from build123d import *

# Parameters (mm, degrees)
BOSS_EXTRUDE1_DEPTH     = 40
SKETCH2_W               = 26
SKETCH2_H               = 6
CUT_EXTRUDE1_DEPTH      = 243.400412541
CUT_EXTRUDE1_DEPTH_BACK = 243.400412541
SKETCH4_R               = 2.5
CUT_EXTRUDE3_START      = 7.142108
SKETCH7_R               = 5
CUT_EXTRUDE3_DEPTH      = 54.857892


with BuildPart() as part:
    # Sketch1 → Boss-Extrude1 (new body)
    with BuildSketch(Plane.XY):
        with BuildLine():
            Line((0, 0), (228.6, 0))
            Line((228.6, 0), (228.6, 70))
            ThreePointArc((228.6, 70), (114.3, 23.006536612), (0, 70))
            Line((0, 70), (0, 0))
        make_face()
    extrude(amount=BOSS_EXTRUDE1_DEPTH)

    # Sketch2 → Cut-Revolve1 (revolve, cut)
    with BuildSketch(Plane(origin=(114.3, 0, 0), x_dir=(0, 0, -1), z_dir=(1, 0, 0))):
        with Locations((-20, 12.006536612)):
            Rectangle(SKETCH2_W, SKETCH2_H)
    revolve(axis=Axis((114.3, 185.506536612, 40), (0, 0, 1)), mode=Mode.SUBTRACT)

    # Sketch4 → Cut-Extrude1 (cut, two sides: drawn at the far end of the back side and taken through both)
    with BuildSketch(Plane.XZ.offset(-CUT_EXTRUDE1_DEPTH_BACK)):
        with Locations(Location((12.7, 20, 0), (0, 0, 270))):
            Circle(SKETCH4_R)
        with Locations(Location((215.9, 20, 0), (0, 0, 270))):
            Circle(SKETCH4_R)
    extrude(amount=CUT_EXTRUDE1_DEPTH + CUT_EXTRUDE1_DEPTH_BACK, mode=Mode.SUBTRACT)

    # Sketch7 → Cut-Extrude3 (cut)
    with BuildSketch(Plane(origin=(0, 70, 0), x_dir=(-1, 0, 0), z_dir=(0, -1, 0)).offset(CUT_EXTRUDE3_START)):
        with Locations(Location((-215.9, -20, 0), (0, 0, 270))):
            Circle(SKETCH7_R)
        with Locations(Location((-12.7, -20, 0), (0, 0, 270))):
            Circle(SKETCH7_R)
    extrude(amount=CUT_EXTRUDE3_DEPTH, mode=Mode.SUBTRACT)

    # Sketch9 → Cut-Revolve3 (revolve, cut)
    with BuildSketch(Plane(origin=(114.3, 0, 0), x_dir=(0, 0, -1), z_dir=(1, 0, 0))):
        Polygon((0, 18.806536612), (0, 23.006536612), (-40, 23.006536612), (-40, 4.806536612), (-2.8, 4.806536612), (-2.8, 9.206536612), (-6.8, 9.206536612), (-6.8, 15.206536612), (-36.8, 15.206536612), (-36.8, 18.806536612), align=None)
    revolve(axis=Axis((114.3, 185.506536612, 40), (0, 0, 1)), mode=Mode.SUBTRACT)


solid = part.part
Verification items for the finished model (mm, model axes). A direction names the side the tool comes from. Coordinates: 2 decimals unless noted, no trailing zeros. Write each loop counter-clockwise with the first axis right and the second up, starting at its lowest first coordinate (ties: lowest second). Pieces come first, ordered by that corner, then holes. Notation, with made-up numbers: (27.25, 24) -> (83.25, 24) arc R12 ccw to (83.25, 30) -> close; hole circle Ø11 at (-32, -26). An arc over 180 degrees is marked (long way). One line per item, written item: value. Start each with the question number.
Q1. Mould release check, pull along X, two halves, no side actions. Record for faces 6 (the flat face through (228.6, 25, 20)), 7 (the cylindrical face through (112.559, 9.215, 4.828)), 8 (the flat face through (113, 0, 20)): pulls with the +X half, pulls with the -X half, needs draft (parallel to the pull), parting line crosses it, or undercut.
Q2. Go/stop test with flat-tipped pins: P1, Ø5, axis at x = 145, z = 35, coming from the -Y side; P2, Ø4.5, axis at x = 215.9, z = 20, coming from the -Y side; P3, Ø11.5, axis at x = 215.9, z = 20, coming from the +Y side; P4, Ø6, axis at x = 12.7, z = 20, coming from the +Y side. Record where each tip stops, or that it passes through.
Q3. Access from +Z, -Z, +X, -X, +Y, -Y to the whole of each face (thin tool, end or side, straight path). Record for faces 1 (the flat face through (115, 7, 2.8)), 2 (the flat face through (113, 18, 0)), 3 (the flat face through (114, 3, 40)), 4 (the flat face through (115, 18, 36.8)), 5 (the flat face through (10, 8, 21)).
Q4. Thickness scan on L1, parallel to X at y = 2, z = 20; L2, parallel to Z at x = 215.9, y = 5.75; L3, parallel to X at y = 39, z = 20. Record the ranges inside material, lowest first. Write a range as from..to.
Q5. Cross-section at B-B on z = 27.5. Enter the section's corners in (x, y), and give its area (3 significant figures).
Q6. Cross-section at A-A on y = 29. Enter the section's corners in (x, z), and give its area (3 significant figures).
Q7. Cross-section at D-D on x = 57. Enter the section's corners in (y, z), and give its area (3 significant figures).
Q8. Cross-section at C-C on x = 12.7. Enter the section's corners in (y, z), and give its area (3 significant figures).
Checked values:
1. face 6: pulls with the +X half
1. face 7: undercut
1. face 8: needs draft
2. P1: stops at y = 0
2. P2: passes through
2. P3: stops at y = 57.97
2. P4: stops at y = 8
3. face 1: +Z
3. face 2: -Z, +X, -X, +Y, -Y
3. face 3: +Z, +X, -X, +Y, -Y
3. face 4: +Z, +Y
3. face 5: +Y
4. L1: x = 0..10.2, 15.2..213.4, 218.4..228.6
4. L2: z = 0..17.5, 22.5..40
4. L3: x = 0..7.7, 27.48..34.77, 193.83..201.12, 220.9..228.6
5. outline: (0, 0) -> (228.6, 0) -> (228.6, 45.55) arc R180.7 cw to (0, 45.55) -> close; (0, 59.26) arc R170.3 ccw to (228.6, 59.26) -> (228.6, 64.16) arc R166.7 cw to (0, 64.16) -> close
5. area: 4,950 mm²
6. outline: (0, 0) -> (56.9, 0) -> (56.9, 36.8) -> (47.16, 36.8) -> (47.16, 6.8) -> (33.14, 6.8) -> (33.14, 2.8) -> (23.98, 2.8) -> (23.98, 40) -> (0, 40) -> close; (171.7, 0) -> (228.6, 0) -> (228.6, 40) -> (204.62, 40) -> (204.62, 2.8) -> (195.46, 2.8) -> (195.46, 6.8) -> (181.44, 6.8) -> (181.44, 36.8) -> (171.7, 36.8) -> close; hole circle Ø10 at (12.7, 20); hole circle Ø10 at (215.9, 20)
6. area: 2,720 mm²
7. outline: (0, 0) -> (28.96, 0) -> (28.96, 36.8) -> (25.14, 36.8) -> (25.14, 6.8) -> (18.78, 6.8) -> (18.78, 2.8) -> (14.13, 2.8) -> (14.13, 40) -> (0, 40) -> close
7. area: 762 mm²
8. outline: (0, 0) -> (53.35, 0) -> (53.35, 15) -> (48.83, 15) -> (48.83, 6.8) -> (41.43, 6.8) -> (41.43, 2.8) -> (36.07, 2.8) -> (36.07, 15) -> (8, 15) -> (8, 17.5) -> (0, 17.5) -> close; (0, 22.5) -> (8, 22.5) -> (8, 25) -> (36.07, 25) -> (36.07, 40) -> (0, 40) -> close; (48.83, 25) -> (53.35, 25) -> (53.35, 36.8) -> (48.83, 36.8) -> close
8. area: 1,310 mm²
